from build123d import *

# Parameters (mm, degrees)
SKETCH2_W           = 256
SKETCH2_H           = 186
BOSS_EXTRUDE1_DEPTH = 3
SKETCH3_R           = 1.6
CUT_EXTRUDE1_DEPTH  = 4
SKETCH4_W           = 56
SKETCH4_H           = 105.9
CUT_EXTRUDE2_DEPTH  = 4
SKETCH5_R           = 1.5
CUT_EXTRUDE3_DEPTH  = 4


with BuildPart() as part:
    # Sketch2 → Boss-Extrude1 (new body)
    with BuildSketch(Plane.XY):
        with Locations((128, 93)):
            Rectangle(SKETCH2_W, SKETCH2_H)
    extrude(amount=BOSS_EXTRUDE1_DEPTH)

    # Sketch3 → Cut-Extrude1 (cut, through all)
    with BuildSketch(Plane.XY.offset(3)):
        with Locations((6, 180)):
            Circle(SKETCH3_R)
        with Locations((128, 180)):
            Circle(SKETCH3_R)
        with Locations((6, 6)):
            Circle(SKETCH3_R)
        with Locations((250, 176)):
            Circle(SKETCH3_R)
        with Locations((250, 10)):
            Circle(SKETCH3_R)
        with Locations((158, 6)):
            Circle(SKETCH3_R)
    extrude(amount=-CUT_EXTRUDE1_DEPTH, mode=Mode.SUBTRACT)

    # Sketch4 → Cut-Extrude2 (cut, through all)
    with BuildSketch(Plane.XY.offset(3)):
        with Locations((121, 59.75)):
            Rectangle(SKETCH4_W, SKETCH4_H)
    extrude(amount=-CUT_EXTRUDE2_DEPTH, mode=Mode.SUBTRACT)

    # Sketch5 → Cut-Extrude3 (cut, through all)
    with BuildSketch(Plane.XY.offset(3)):
        with Locations((173, 105)):
            Circle(SKETCH5_R)
        with Locations((167, 105)):
            Circle(SKETCH5_R)
        with Locations((161, 105)):
            Circle(SKETCH5_R)
        with Locations((155, 105)):
            Circle(SKETCH5_R)
        with Locations((167, 99)):
            Circle(SKETCH5_R)
        with Locations((161, 99)):
            Circle(SKETCH5_R)
        with Locations((155, 99)):
            Circle(SKETCH5_R)
        with Locations((167, 93)):
            Circle(SKETCH5_R)
        with Locations((161, 93)):
            Circle(SKETCH5_R)
        with Locations((155, 93)):
            Circle(SKETCH5_R)
        with Locations((167, 87)):
            Circle(SKETCH5_R)
        with Locations((161, 87)):
            Circle(SKETCH5_R)
        with Locations((155, 87)):
            Circle(SKETCH5_R)
        with Locations((167, 81)):
            Circle(SKETCH5_R)
        with Locations((161, 81)):
            Circle(SKETCH5_R)
        with Locations((155, 81)):
            Circle(SKETCH5_R)
        with Locations((167, 75)):
            Circle(SKETCH5_R)
        with Locations((161, 75)):
            Circle(SKETCH5_R)
        with Locations((155, 75)):
            Circle(SKETCH5_R)
        with Locations((167, 69)):
            Circle(SKETCH5_R)
        with Locations((161, 69)):
            Circle(SKETCH5_R)
        with Locations((155, 69)):
            Circle(SKETCH5_R)
        with Locations((167, 63)):
            Circle(SKETCH5_R)
        with Locations((161, 63)):
            Circle(SKETCH5_R)
        with Locations((155, 63)):
            Circle(SKETCH5_R)
        with Locations((167, 57)):
            Circle(SKETCH5_R)
        with Locations((161, 57)):
            Circle(SKETCH5_R)
        with Locations((155, 57)):
            Circle(SKETCH5_R)
        with Locations((167, 51)):
            Circle(SKETCH5_R)
        with Locations((161, 51)):
            Circle(SKETCH5_R)
        with Locations((155, 51)):
            Circle(SKETCH5_R)
        with Locations((167, 45)):
            Circle(SKETCH5_R)
        with Locations((161, 45)):
            Circle(SKETCH5_R)
        with Locations((155, 45)):
            Circle(SKETCH5_R)
        with Locations((167, 39)):
            Circle(SKETCH5_R)
        with Locations((161, 39)):
            Circle(SKETCH5_R)
        with Locations((155, 39)):
            Circle(SKETCH5_R)
        with Locations((167, 33)):
            Circle(SKETCH5_R)
        with Locations((161, 33)):
            Circle(SKETCH5_R)
        with Locations((155, 33)):
            Circle(SKETCH5_R)
        with Locations((167, 27)):
            Circle(SKETCH5_R)
        with Locations((161, 27)):
            Circle(SKETCH5_R)
        with Locations((155, 27)):
            Circle(SKETCH5_R)
        with Locations((167, 21)):
            Circle(SKETCH5_R)
        with Locations((161, 21)):
            Circle(SKETCH5_R)
        with Locations((155, 21)):
            Circle(SKETCH5_R)
        with Locations((167, 15)):
            Circle(SKETCH5_R)
        with Locations((161, 15)):
            Circle(SKETCH5_R)
        with Locations((155, 15)):
            Circle(SKETCH5_R)
        with Locations((173, 99)):
            Circle(SKETCH5_R)
        with Locations((173, 93)):
            Circle(SKETCH5_R)
        with Locations((173, 87)):
            Circle(SKETCH5_R)
        with Locations((173, 81)):
            Circle(SKETCH5_R)
        with Locations((173, 75)):
            Circle(SKETCH5_R)
        with Locations((173, 69)):
            Circle(SKETCH5_R)
        with Locations((173, 63)):
            Circle(SKETCH5_R)
        with Locations((173, 57)):
            Circle(SKETCH5_R)
        with Locations((173, 51)):
            Circle(SKETCH5_R)
        with Locations((173, 45)):
            Circle(SKETCH5_R)
        with Locations((173, 39)):
            Circle(SKETCH5_R)
        with Locations((173, 33)):
            Circle(SKETCH5_R)
        with Locations((173, 27)):
            Circle(SKETCH5_R)
        with Locations((173, 21)):
            Circle(SKETCH5_R)
        with Locations((173, 15)):
            Circle(SKETCH5_R)
    extrude(amount=-CUT_EXTRUDE3_DEPTH, mode=Mode.SUBTRACT)


solid = part.part
For this review, take the finished solid that the model builds, in its own axes (mm). Give positions to 0.01 mm unless a question says otherwise; leave off trailing zeros. Loops run counter-clockwise (first coordinate to the right, second up) from the corner with the lowest first, then second, coordinate; pieces in that order, holes last. Notation, with made-up numbers: M 21,79 L 62,79 A25 cw 62,99 Z; hole C 26.25,-1.75 d8. An arc over 180 degrees is marked long. Answer as a JSON object with one key per item and string values. Group by question number.
Q1. Add section B-B on z = 1.05. Give the number of separate pieces and of enclosed holes in the cut face, and give its area (3 significant figures).
Q2. Add section A-A on x = 109.5. Give the boundary of the cut face in (y, z).
Q3. For probe 1 along X at (y, z) = (93, 0.9); probe 2 along X at (y, z) = (35, 2.4); probe 3 along X at (y, z) = (106, 1.65), list the stretches that pass through material, from the lowest coordinate up. Write a range as [from, to].
Checked values:
{
 "1": {"separate pieces": "1", "enclosed holes": "71", "area": "41,200 mm²"},
 "2": {"outline": "M 0,0 L 6.8,0 L 6.8,3 L 0,3 Z; M 112.7,0 L 186,0 L 186,3 L 112.7,3 Z"},
 "3": {"probe 1": "[0, 93], [149, 153.5], [156.5, 159.5], [162.5, 165.5], [168.5, 171.5], [174.5, 256]", "probe 2": "[0, 93], [149, 256]", "probe 3": "[0, 93], [149, 153.88], [156.12, 159.88], [162.12, 165.88], [168.12, 171.88], [174.12, 256]"}
}
